Geometry: see drawing. Coordinates: mm, zero at the bounding-box minimum. Coordinates: 2 decimals unless noted, no trailing zeros. Order: outer loops, then holes, each group sorted by start corner. A loop starts at its lowest first (then second) coordinate and runs counter-clockwise, first axis right, second up.
Item 1: Section C-C on z = 85. Return the cut outline in (x, y), then the cut area to 3 significant figures.
Item 2: Section B-B on x = 152.5. Return the cut outline in (y, z) (1 decimal).
Item 3: Contact query for flat-ended pins moving along their axis: P1, Ø5, axis at y = 6.5, z = 24.5, coming from the -X side; P2, Ø10, axis at x = 92.5, y = 5, coming from the +Z side; P3, Ø6, axis at y = 13, z = 70, coming from the -X side; P4, Ø12, axis at x = 92.5, z = 34, coming from the -Y side. Output: stop coordinate, or through.
Item 4: Section A-A on y = 12. Return the cut outline in (x, z) (1 decimal).
Item 5: Ray query, line 1 (X direction, y = 2, z = 42.5); line 2 (X direction, y = 15.5, z = 41) (1 decimal); line 3 (Z direction, x = 164.5, y = 24) (1 decimal). Return the intervals inside material, ascending.
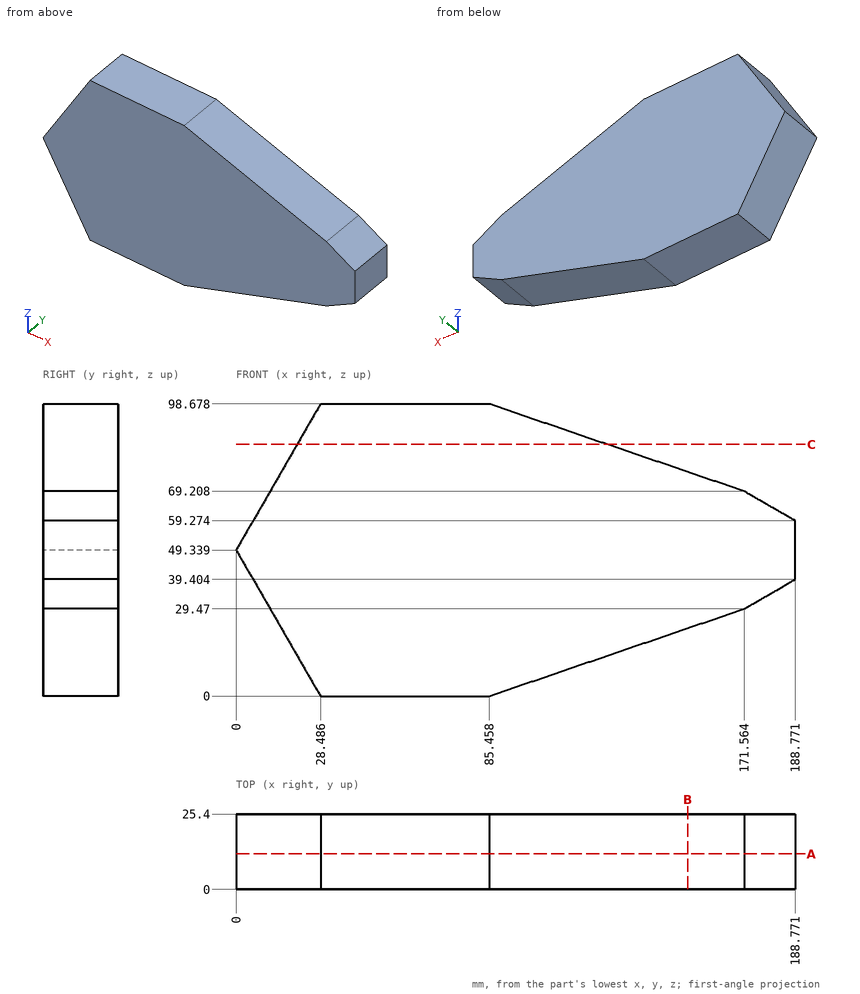
Answer list:
1. outline: (20.59, 0) - (125.42, 0) - (125.42, 25.4) - (20.59, 25.4) - close
1. area: 2,660 mm2
2. outline: (0, 22.9) - (25.4, 22.9) - (25.4, 75.7) - (0, 75.7) - close
3. P1: stops at x = 12.9
3. P2: stops at z = 97.98
3. P3: stops at x = 10.2
3. P4: stops at y = 0
4. outline: (0, 49.3) - (28.5, 0) - (85.5, 0) - (171.6, 29.5) - (188.8, 39.4) - (188.8, 59.3) - (171.6, 69.2) - (85.5, 98.7) - (28.5, 98.7) - close
5. line 1: x = 3.95 to 188.77
5. line 2: x = 4.8 to 188.8
5. line 3: z = 27.1 to 71.6
